from build123d import *

# Parameters (mm, degrees)
F0_W     = 4
F0_H     = 16
F1_DEPTH = 1
F0_W_2   = 1.4000003636
F0_H_2   = 11.8
F0_H_3   = 2
F2_DEPTH = 7.4
F3_DEPTH = 2.6
F4_DEPTH = 4.5
F5_DEPTH = 4


# Not quite as in the source:
# - ends of sketch curves that miss each other by under 0.0002 mm in the source are joined
# - a feature names something its author has since deleted; it is built from what else it names


with BuildPart() as f1:
    # F0 (on Top) → F1 (new body)
    with BuildSketch(Plane.XY):
        Polygon((-46.6793118417, -34.5732776225), (-46.6793118417, -35.6732776225), (9.7206891477, -35.6732776225), (9.7206891477, -37.6732772589), (19.7206891477, -37.6732772589), (19.7206891477, -35.5732776225), (29.4207941621, -35.5732776225), (29.4207941621, -34.5732776225), (31.9206877947, -34.5732776225), (31.9206877947, -26.0732776225), (29.4206877947, -26.0732776225), (29.4206877947, -24.5732776225), (21.4206877947, -24.5732776225), (21.4206877947, -12.7732776225), (21.4206877947, -10.7732776225), (29.4206877947, -10.7732776225), (29.4206877947, 0.2267237306), (-46.6793118417, 0.2267237306), (-46.6793118417, -15.5122037977), (-37.1793118417, -15.5122037977), (-37.1793118417, -18.5732776225), (-37.1793118417, -34.5732776225), (-41.1793118417, -34.5732776225), (-41.1793118417, -18.5732776225), (-46.6793118417, -18.5732776225), (-49.1793118417, -18.5732776225), (-49.1793118417, -34.5732776225), align=None)
        Polygon((-49.1793118417, 2.7267237306), (-49.1793118417, -18.5732776225), (-46.6793118417, -18.5732776225), (-46.6793118417, -15.5122037977), (-46.6793118417, 0.2267237306), (29.4206877947, 0.2267237306), (29.4206877947, -10.7732776225), (31.9206877947, -10.7732776225), (31.9206877947, 2.7267237306), align=None)
        Polygon((-50.6793118417, -1.5732776225), (-50.6793118417, -18.5732776225), (-49.1793118417, -18.5732776225), (-49.1793118417, 2.7267237306), (31.9206877947, 2.7267237306), (31.9206877947, -10.7732776225), (33.3206881583, -10.7732776225), (33.3206881583, 6.4267223775), (30.3206881583, 6.4267223775), (-50.6793118417, 6.4267223775), align=None)
        Polygon((-46.6793118417, -35.6732776225), (-46.6793118417, -38.0732776225), (7.2206891477, -38.0732776225), (7.2206891477, -40.1732772589), (22.2206891477, -40.1732772589), (22.2206891477, -38.0732776225), (29.4207941621, -38.0732776225), (31.9206877947, -38.0732776225), (31.9206877947, -34.5732776225), (29.4207941621, -34.5732776225), (29.4207941621, -35.5732776225), (19.7206891477, -35.5732776225), (19.7206891477, -37.6732772589), (9.7206891477, -37.6732772589), (9.7206891477, -35.6732776225), align=None)
        Polygon((-50.6793118417, -38.0732776225), (-50.6793118417, -41.5732776225), (30.3206881583, -41.5732776225), (33.3206881583, -41.5732776225), (33.3206349746, -38.0732776225), (31.9206877947, -38.0732776225), (29.4207941621, -38.0732776225), (22.2206891477, -38.0732776225), (22.2206891477, -40.1732772589), (7.2206891477, -40.1732772589), (7.2206891477, -38.0732776225), (-46.6793118417, -38.0732776225), (-50.1793118417, -38.0732776225), align=None)
        Polygon((31.9206877947, -26.0732776225), (33.3206881583, -26.0732776225), (33.3206881583, -24.5732776225), (31.9206877947, -24.5732776225), (31.9206877947, -25.7732776225), align=None)
        Polygon((33.3205817909, -34.5732776225), (33.3206349746, -38.0732776225), (33.3206881583, -26.0732776225), (31.9206877947, -26.0732776225), (31.9206877947, -34.5732776225), align=None)
        Polygon((31.9206877947, -38.0732776225), (33.3206349746, -38.0732776225), (33.3205817909, -34.5732776225), (31.9206877947, -34.5732776225), align=None)
        Polygon((-50.6793118417, -18.5732776225), (-50.6793118417, -34.5732776225), (-50.1793118417, -34.5732776225), (-49.1793118417, -34.5732776225), (-49.1793118417, -18.5732776225), align=None)
        Polygon((-50.1793118417, -34.5732776225), (-50.1793118417, -38.0732776225), (-46.6793118417, -38.0732776225), (-46.6793118417, -35.6732776225), (-46.6793118417, -34.5732776225), (-49.1793118417, -34.5732776225), align=None)
        Polygon((-50.6793118417, -35.5732776225), (-50.6793118417, -38.0732776225), (-50.1793118417, -38.0732776225), (-50.1793118417, -34.5732776225), (-50.6793118417, -34.5732776225), align=None)
        with Locations((-39.1793118417, -26.5732776225)):
            Rectangle(F0_W, F0_H)
        Polygon((-46.6793118417, -15.5122037977), (-46.6793118417, -18.5732776225), (-41.1793118417, -18.5732776225), (-37.1793118417, -18.5732776225), (-37.1793118417, -15.5122037977), align=None)
        Polygon((29.4206877947, -26.0732776225), (31.9206877947, -26.0732776225), (31.9206877947, -25.7732776225), (31.9206877947, -24.5732776225), (29.4206877947, -24.5732776225), align=None)
    extrude(amount=-F1_DEPTH)

    # F0 (on Top) → F2 (join)
    with BuildSketch(Plane.XY):
        Polygon((-50.6793118417, -38.0732776225), (-50.6793118417, -41.5732776225), (30.3206881583, -41.5732776225), (33.3206881583, -41.5732776225), (33.3206349746, -38.0732776225), (31.9206877947, -38.0732776225), (29.4207941621, -38.0732776225), (22.2206891477, -38.0732776225), (22.2206891477, -40.1732772589), (7.2206891477, -40.1732772589), (7.2206891477, -38.0732776225), (-46.6793118417, -38.0732776225), (-50.1793118417, -38.0732776225), align=None)
        Polygon((-50.6793118417, -1.5732776225), (-50.6793118417, -18.5732776225), (-49.1793118417, -18.5732776225), (-49.1793118417, 2.7267237306), (31.9206877947, 2.7267237306), (31.9206877947, -10.7732776225), (33.3206881583, -10.7732776225), (33.3206881583, 6.4267223775), (30.3206881583, 6.4267223775), (-50.6793118417, 6.4267223775), align=None)
        Polygon((31.9206877947, -26.0732776225), (33.3206881583, -26.0732776225), (33.3206881583, -24.5732776225), (31.9206877947, -24.5732776225), (31.9206877947, -25.7732776225), align=None)
        Polygon((33.3205817909, -34.5732776225), (33.3206349746, -38.0732776225), (33.3206881583, -26.0732776225), (31.9206877947, -26.0732776225), (31.9206877947, -34.5732776225), align=None)
        Polygon((31.9206877947, -38.0732776225), (33.3206349746, -38.0732776225), (33.3205817909, -34.5732776225), (31.9206877947, -34.5732776225), align=None)
        Polygon((-50.6793118417, -35.5732776225), (-50.6793118417, -38.0732776225), (-50.1793118417, -38.0732776225), (-50.1793118417, -34.5732776225), (-50.6793118417, -34.5732776225), align=None)
        with Locations((32.6206879765, -18.6732776225)):
            Rectangle(F0_W_2, F0_H_2)
        with Locations((32.6206879765, -11.7732776225)):
            Rectangle(F0_W_2, F0_H_3)
    extrude(amount=F2_DEPTH)

    # F0 (on Top) → F3 (join)
    with BuildSketch(Plane.XY):
        Polygon((-50.6793118417, -18.5732776225), (-50.6793118417, -34.5732776225), (-50.1793118417, -34.5732776225), (-49.1793118417, -34.5732776225), (-49.1793118417, -18.5732776225), align=None)
    extrude(amount=F3_DEPTH)

    # F0 (on Top) → F4 (join)
    with BuildSketch(Plane.XY):
        with Locations((-39.1793118417, -26.5732776225)):
            Rectangle(F0_W, F0_H)
        Polygon((-46.6793118417, -15.5122037977), (-46.6793118417, -18.5732776225), (-41.1793118417, -18.5732776225), (-37.1793118417, -18.5732776225), (-37.1793118417, -15.5122037977), align=None)
    extrude(amount=F4_DEPTH)

    # F0 (on Top) → F5 (cut)
    with BuildSketch(Plane.XY):
        with Locations((32.6206879765, -18.6732776225)):
            Rectangle(F0_W_2, F0_H_2)
        with Locations((32.6206879765, -11.7732776225)):
            Rectangle(F0_W_2, F0_H_3)
    extrude(amount=F5_DEPTH, mode=Mode.SUBTRACT)


solid = f1.part
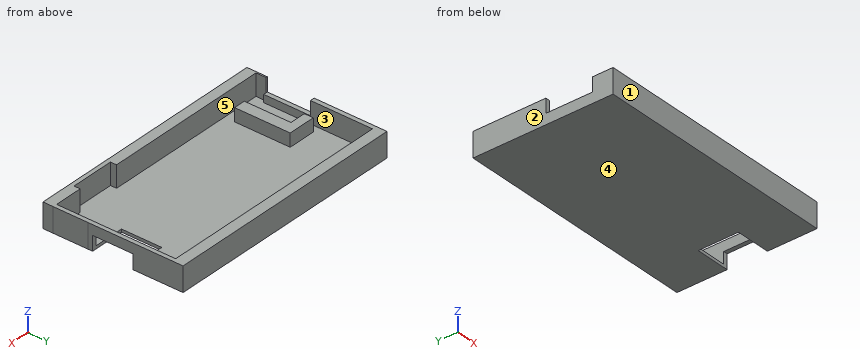
Build history of the part. All positions in model axes, mm. Face numbers are marked on the shaded views. A direction names the side the tool comes from. Round coordinates to 2 decimals unless told otherwise and drop trailing zeros. Write each loop counter-clockwise with the first axis right and the second up, starting at its lowest first coordinate (ties: lowest second). Pieces come first, ordered by that corner, then holes. Notation, with made-up numbers: (66.25, -19.75) - (104.25, -19.75) arc R23 ccw to (104.25, 3.25) - close; hole circle Ø9 at (42.5, 74). An arc over 180 degrees is marked (long way). Use CSV: the item, a comma, the result in double quotes.
(1) Mould opens along Y. For the marked faces 1, 2 and 3 say: pulls with the +Y half, pulls with the -Y half, needs draft (parallel to the pull), parting line crosses it, or undercut.
Response:
face 1,"pulls with the -Y half"
face 2,"needs draft"
face 3,"undercut"
(2) 3-axis set-ups, long thin cutter, end or side, ignore diameter. For the marked faces 4 and 5: which of +Z, -Z, +X, -X, +Y, -Y reach the whole face in a straight line?
Response:
face 4,"-Z, +X, -X, +Y, -Y"
face 5,"+Z"
(3) Band-saw the part on B-B (y = -14.5). Write the cut outline in (x, z), plus the area to 3 significant figures.
Response:
outline,"(-50.68, -1) - (21.42, -1) - (21.42, 0) - (-49.18, 0) - (-49.18, 7.4) - (-50.68, 7.4) - close; (31.92, 4) - (33.32, 4) - (33.32, 7.4) - (31.92, 7.4) - close"
area,"88.0 mm²"
(4) Wall check: line 1 (Y direction, x = -40.5, z = 0.75); line 2 (X direction, y = -5, z = 6.25); line 3 (Y direction, x = -3, z = 1). Give the ranges that are in metal, low to high.
Response:
line 1,"-41.57 to -38.07, -34.57 to -15.51, 2.73 to 6.43"
line 2,"-50.68 to -49.18, 31.92 to 33.32"
line 3,"-41.57 to -38.07, 2.73 to 6.43"
(5) Band-saw the part on C-C (z = 6). Write the cut outline in (x, y), plus the area to 3 significant figures.
Response:
outline,"(-50.68, -41.57) - (33.32, -41.57) - (33.32, -38.07) - (33.32, -26.07) - (33.32, 6.43) - (-50.68, 6.43) - (-50.68, -18.57) - (-49.18, -18.57) - (-49.18, 2.73) - (31.92, 2.73) - (31.92, -38.07) - (22.22, -38.07) - (22.22, -40.17) - (7.22, -40.17) - (7.22, -38.07) - (-50.18, -38.07) - (-50.18, -34.57) - (-50.68, -34.57) - close"
area,"664 mm²"
(6) Band-saw the part on D-D (x = -45). Write the cut outline in (y, z), plus the area to 3 significant figures.
Response:
outline,"(-41.57, -1) - (6.43, -1) - (6.43, 7.4) - (2.73, 7.4) - (2.73, 0) - (-15.51, 0) - (-15.51, 4.5) - (-18.57, 4.5) - (-18.57, 0) - (-38.07, 0) - (-38.07, 7.4) - (-41.57, 7.4) - close"
area,"115 mm²"
(7) Pin check, flat tips, straight feed: P1, Ø1.5, axis at x = -32, y = 0, coming from the +Z side; P2, Ø1.2, axis at x = -50.5, y = -28, coming from the +Z side; P3, Ø3, axis at y = -20, z = 5, coming from the -X side. Stop position of each tip, or through.
Response:
P1,"z = 0"
P2,"z = 2.6"
P3,"x = -50.68"
(8) Band-saw the part on A-A (z = 1.75). Write the cut outline in (x, y).
Response:
outline,"(-50.68, -41.57) - (33.32, -41.57) - (33.32, -38.07) - (33.32, -26.07) - (33.32, -24.57) - (31.92, -24.57) - (31.92, -38.07) - (22.22, -38.07) - (22.22, -40.17) - (7.22, -40.17) - (7.22, -38.07) - (-50.18, -38.07) - (-50.18, -34.57) - (-49.18, -34.57) - (-49.18, 2.73) - (31.92, 2.73) - (31.92, -10.77) - (33.32, -10.77) - (33.32, 6.43) - (-50.68, 6.43) - close; (-46.68, -18.57) - (-41.18, -18.57) - (-41.18, -34.57) - (-37.18, -34.57) - (-37.18, -15.51) - (-46.68, -15.51) - close"
